CAD build for the part. Positions are in the model's coordinates, mm. Round coordinates to 2 decimals unless told otherwise and drop trailing zeros. Loops run counter-clockwise (first coordinate to the right, second up) from the corner with the lowest first, then second, coordinate; pieces in that order, holes last. Notation, with made-up numbers: M 89.5,-14.5 L 131.5,-14.5 A18 cw 131.5,14.5 Z; hole C -15.75,59.25 d2. An arc over 180 degrees is marked long. Use one line per item in the form item = value.
from build123d import *

# Parameters (mm, degrees)
BOSS_EXTRUDE3_DEPTH = 30
BOSS_EXTRUDE4_DEPTH = 10
SKETCH4_W           = 80
SKETCH4_H           = 5
BOSS_EXTRUDE5_DEPTH = 5


with BuildPart() as part:
    # Sketch1 → Boss-Extrude3 (new body)
    with BuildSketch(Plane(origin=(0, 0, 0), x_dir=(0, 0, -1), z_dir=(1, 0, 0))):
        with BuildLine():
            Line((-50, 0), (-45, 0))
            ThreePointArc((-45, 0), (0, 45), (45, 0))
            Line((45, 0), (50, 0))
            ThreePointArc((50, 0), (0, 50), (-50, 0))
        make_face()
    extrude(amount=BOSS_EXTRUDE3_DEPTH)

    # Sketch3 → Boss-Extrude4 (add)
    with BuildSketch(Plane(origin=(30, 0, 0), x_dir=(0, 0, -1), z_dir=(1, 0, 0))):
        with BuildLine():
            Line((-5.226423163, 49.726094768), (-4.703780847, 44.753485292))
            ThreePointArc((-4.703780847, 44.753485292), (-2.355118031, 44.938329064), (0, 45))
            Line((0, 45), (0, 50))
            ThreePointArc((0, 50), (-2.616797812, 49.931476738), (-5.226423163, 49.726094768))
        make_face()
        with BuildLine():
            ThreePointArc((0, 45), (2.355118031, 44.938329064), (4.703780847, 44.753485292))
            Line((4.703780847, 44.753485292), (5.226423163, 49.726094768))
            ThreePointArc((5.226423163, 49.726094768), (2.616797812, 49.931476738), (0, 50))
            Line((0, 50), (0, 45))
        make_face()
    extrude(amount=BOSS_EXTRUDE4_DEPTH)

    # Mirror3: part across plane


with BuildPart() as part_1:
    add(part.part)
    add(part.part.mirror(Plane(origin=(40, 0, 0), x_dir=(0, 0, 1), z_dir=(1, 0, 0))))

    # Sketch4 → Boss-Extrude5 (add)
    with BuildSketch(Plane.XZ):
        with Locations((40, 47.5)):
            Rectangle(SKETCH4_W, SKETCH4_H)
        with Locations((40, -47.5)):
            Rectangle(SKETCH4_W, SKETCH4_H)
    extrude(amount=BOSS_EXTRUDE5_DEPTH)


solid = part_1.part
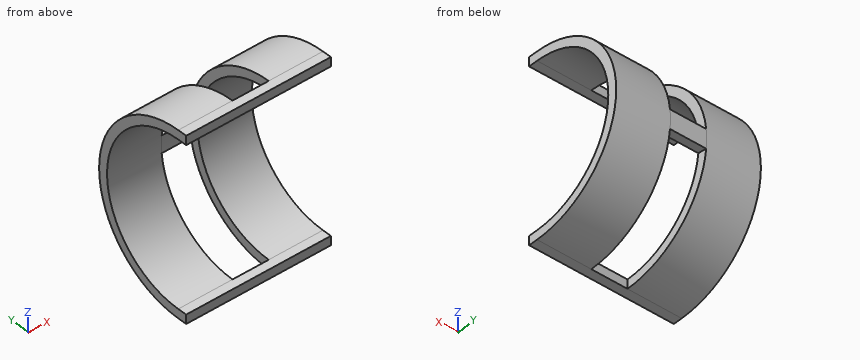
1. Drop flat-ended pins along their axis: P1, Ø4, axis at x = 59.5, z = -9.5, coming from the -Y side; P2, Ø12, axis at x = 19, z = 25, coming from the +Y side; P3, Ø10, axis at x = 9, z = -23.5, coming from the +Y side. Give the stop position or say it passes through.
Completed:
P1 = 43.51
P2 = 46.25
P3 = 46.45
2. Cut at C-C on y = 30. Write the cut outline in (x, z), and give its area (3 significant figures).
Completed:
outline = M 0,-40 L 30,-40 L 30,-33.54 L 0,-33.54 Z; M 0,33.54 L 30,33.54 L 30,40 L 0,40 Z; M 50,-40 L 80,-40 L 80,-33.54 L 50,-33.54 Z; M 50,33.54 L 80,33.54 L 80,40 L 50,40 Z
area = 775 mm2
3. Cut at A-A on x = 38.5. Write the cut outline in (y, z).
Completed:
outline = M -5,-50 L 0,-50 L 0,-45 L -5,-45 Z; M -5,45 L 0,45 L 0,50 L -5,50 Z; M 44.75,-4.7 L 49.73,-5.23 A50 ccw 49.73,5.23 L 44.75,4.7 A45 cw Z
4. Cut at D-D on x = 19. Write the cut outline in (y, z), and give its area (3 significant figures).
Completed:
outline = M -5,-50 L 0,-50 A50 ccw 0,50 L -5,50 L -5,45 L 0,45 A45 cw 0,-45 L -5,-45 Z
area = 796 mm2
5. Probe line 1 along X through (y, z) = (43, 17.5); line 2 along Z through (x, y) = (67, 12); line 3 along Z through (x, y) = (11, 35). List the from-to ranges inside material, lowest first. Write a range as from..to.
Completed:
line_1 = 0..30, 50..80
line_2 = -48.54..-43.37, 43.37..48.54
line_3 = -35.71..-28.28, 28.28..35.71
6. Cut at B-B on z = -25.5. Write the cut outline in (x, y).
Completed:
outline = M 0,37.08 L 30,37.08 L 30,43.01 L 0,43.01 Z; M 50,37.08 L 80,37.08 L 80,43.01 L 50,43.01 Z
